```python
from build123d import *

# Parameters (mm, degrees)
SKETCH1_W                       = 47.752
SKETCH1_H                       = 69.215
SKETCH1_W_2                     = 42.672
SKETCH1_H_2                     = 64.135
BOSS_EXTRUDE1_DEPTH             = 50.8
BOSS_EXTRUDE2_DEPTH             = 6.35
F_9_64_0_14063_DIAMETER_HOLE1_D = 3.572002
SKETCH11_W                      = 12.7
SKETCH11_H                      = 36.195
CUT_EXTRUDE1_DEPTH              = 6.35
SKETCH12_W                      = 10.16
SKETCH12_H                      = 34.29
CUT_EXTRUDE2_DEPTH              = 6.35


with BuildPart() as part:
    # Sketch1 → Boss-Extrude1 (new body)
    with BuildSketch(Plane(origin=(0, 0, 0), x_dir=(1, 0, 0), z_dir=(0, 1, 0))):
        with Locations((21.336, 32.0675)):
            Rectangle(SKETCH1_W, SKETCH1_H)
        with Locations((21.336, 32.0675)):
            Rectangle(SKETCH1_W_2, SKETCH1_H_2, mode=Mode.SUBTRACT)
    extrude(amount=BOSS_EXTRUDE1_DEPTH)

    # Sketch2 → Boss-Extrude2 (add)
    with BuildSketch(Plane.XZ):
        with BuildLine():
            Line((-5.715, -3.81), (-2.54, -3.81))
            Line((-2.54, -3.81), (-2.54, 2.54))
            Line((-2.54, 2.54), (-5.715, 2.54))
            ThreePointArc((-5.715, 2.54), (-8.89, -0.635), (-5.715, -3.81))
        make_face()
        with BuildLine():
            Line((48.387, -60.325), (45.212, -60.325))
            Line((45.212, -60.325), (45.212, -66.675))
            Line((45.212, -66.675), (48.387, -66.675))
            ThreePointArc((48.387, -66.675), (51.562, -63.5), (48.387, -60.325))
        make_face()
        with BuildLine():
            Line((-2.54, -66.675), (-5.715, -66.675))
            ThreePointArc((-5.715, -66.675), (-8.89, -63.5), (-5.715, -60.325))
            Line((-5.715, -60.325), (-2.54, -60.325))
            Line((-2.54, -60.325), (-2.54, -66.675))
        make_face()
        with BuildLine():
            Line((45.212, 2.54), (48.387, 2.54))
            ThreePointArc((48.387, 2.54), (51.562, -0.635), (48.387, -3.81))
            Line((48.387, -3.81), (45.212, -3.81))
            Line((45.212, -3.81), (45.212, 2.54))
        make_face()
    extrude(amount=-BOSS_EXTRUDE2_DEPTH)

    # 9/64 (0.14063) Diameter Hole1 (through all)
    with Locations(Plane(origin=(0, 6.35, 0), x_dir=(1, 0, 0), z_dir=(0, 1, 0))):
        with Locations((-5.715, 0.635), (-5.715, 63.5), (48.387, 63.5), (48.387, 0.635)):
            Hole(F_9_64_0_14063_DIAMETER_HOLE1_D / 2)

    # Sketch11 → Cut-Extrude1 (cut)
    with BuildSketch(Plane.ZY.offset(2.54)):
        with Locations((-6.985, 32.7025)):
            Rectangle(SKETCH11_W, SKETCH11_H)
    extrude(amount=-CUT_EXTRUDE1_DEPTH, mode=Mode.SUBTRACT)

    # Sketch12 → Cut-Extrude2 (cut)
    with BuildSketch(Plane(origin=(0, 0, -66.675), x_dir=(-1, 0, 0), z_dir=(0, 0, -1))):
        with Locations((-5.588, 33.655)):
            Rectangle(SKETCH12_W, SKETCH12_H)
    extrude(amount=-CUT_EXTRUDE2_DEPTH, mode=Mode.SUBTRACT)


solid = part.part
```
Could you check a few things on this model? Use its own coordinates, in mm. A direction names the side the tool comes from. Coordinates: 2 decimals unless noted, no trailing zeros. Write each loop counter-clockwise with the first axis right and the second up, starting at its lowest first coordinate (ties: lowest second). Pieces come first, ordered by that corner, then holes. Notation, with made-up numbers: (-38, 47) -> (5, 47) arc R9 cw to (5, 62) -> close; hole circle Ø7 at (-18, -13). An arc over 180 degrees is marked (long way). Write item = value, one per line. Start each with the question number.
(1) We'd pull the mould along X, two halves only. Please class faces 4 (the face through (50.17, 3.13, -0.71)), 5 (the face through (-8.89, 3.13, -63.57)), 6 (the face through (22, 25, 2.54)): released by +X, released by -X, zero draft, split by the parting line, or undercut.
(2) I want a section at D-D (y = 10). Please give me the cut outline in (x, z) (3 decimals).
(3) I need wall thicknesses on line 1 (X direction, y = 4.25, z = -63.5); line 2 (Z direction, x = 5, y = 16) (3 decimals); line 3 (X direction, y = 26, z = -40). Which ranges of each line are inside material? Lowest first, please. Write a range as [from, to].
(4) I want a section at C-C (z = -47). Please give me the cut outline in (x, y), plus the area to 3 significant figures.
(5) I want a section at B-B (x = 3.5). Please give me the cut outline in (y, z) (3 decimals).
(6) I want a section at A-A (y = 26.5). Please give me the cut outline in (x, z) (3 decimals).
(7) Will these pins go through, and if not, where does the flat tip stop? pin 1 (4.5 mm diameter, centred on x = -5.715, z = -63.5, fed in from -Y); pin 2 (0.8 mm diameter, centred on x = 5.5, z = -66, fed in from +Y); pin 3 (1.3 mm diameter, centred on y = 31, z = -65, fed in from +X); pin 4 (2 mm diameter, centred on y = 38, z = -66, fed in from -X).
(8) Which directions (+Z, -Z, +X, -X, +Y, -Y) give clear straight access to the entire face, cutting with the end or side of a thin tool? Please do faces 1 (the face through (-1, 14.605, -7)), 2 (the face through (21, 25, 0)), 3 (the face through (-4, 3, -60.325)).
Result set:
q1.face_4 = undercut
q1.face_5 = released by -X
q1.face_6 = zero draft
q2.outline = (-2.54, -66.675) -> (45.212, -66.675) -> (45.212, 2.54) -> (-2.54, 2.54) -> close; hole (0, -64.135) -> (42.672, -64.135) -> (42.672, 0) -> (0, 0) -> close
q3.line_1 = [-8.89, -7.5], [-3.93, 0], [42.67, 46.6], [50.17, 51.56]
q3.line_2 = [-66.675, -64.135], [0, 2.54]
q3.line_3 = [-2.54, 0], [42.67, 45.21]
q4.outline = (-2.54, 0) -> (0, 0) -> (0, 50.8) -> (-2.54, 50.8) -> close; (42.67, 0) -> (45.21, 0) -> (45.21, 50.8) -> (42.67, 50.8) -> close
q4.area = 258 mm2
q5.outline = (0, -66.675) -> (16.51, -66.675) -> (16.51, -64.135) -> (0, -64.135) -> close; (0, 0) -> (50.8, 0) -> (50.8, 2.54) -> (0, 2.54) -> close
q6.outline = (-2.54, -66.675) -> (0.508, -66.675) -> (0.508, -64.135) -> (0, -64.135) -> (0, -13.335) -> (-2.54, -13.335) -> close; (-2.54, -0.635) -> (0, -0.635) -> (0, 0) -> (42.672, 0) -> (42.672, -64.135) -> (10.668, -64.135) -> (10.668, -66.675) -> (45.212, -66.675) -> (45.212, 2.54) -> (-2.54, 2.54) -> close
q7.pin_1 = 0
q7.pin_2 = 16.51
q7.pin_3 = 45.21
q7.pin_4 = -2.54
q8.face_1 = -X, +Y
q8.face_2 = +Y, -Y
q8.face_3 = -X, +Y, -Y
